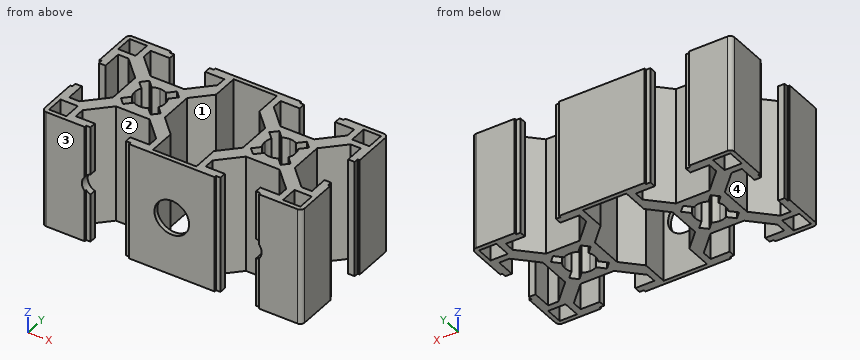
```python
from build123d import *

# Parameters (mm, degrees)
ESBO_O1_W                      = 4
ESBO_O1_H                      = 4
RESSALTO_EXTRUS_O1_DEPTH       = 27
PADR_OCIRCULAR1_COUNT          = 4
PADR_O_LINEAR1_COUNT           = 2
PADR_O_LINEAR1_PITCH           = 30
PADR_O_LINEAR1_COPY_1_SKETCH_W = 4
PADR_O_LINEAR1_COPY_1_SKETCH_H = 4
PADR_O_LINEAR1_COPY_1_DEPTH    = 27
PADR_O_LINEAR1_COPY_2_SKETCH_W = 4
PADR_O_LINEAR1_COPY_2_SKETCH_H = 4
PADR_O_LINEAR1_COPY_2_DEPTH    = 27
PADR_O_LINEAR1_COPY_3_SKETCH_W = 4
PADR_O_LINEAR1_COPY_3_SKETCH_H = 4
PADR_O_LINEAR1_COPY_3_DEPTH    = 27
ESBO_O4_W                      = 10
ESBO_O4_H                      = 28
CORTE_EXTRUS_O1_DEPTH          = 55.580216196
FILETE1_R                      = 1
SKETCH1_R                      = 2.5
SKETCH1_R_2                    = 4
CUT_EXTRUDE1_DEPTH             = 6


with BuildPart() as part:
    # Esboço1 → Ressalto-extrusão1 (new body)
    with BuildSketch(Plane.XY):
        with BuildLine():
            ThreePointArc((-1.664601464, 3.078815026), (-0.858529967, 3.393070335), (0, 3.5))
            Line((0, 3.5), (0, 6))
            Line((0, 6), (-3.878679656, 6))
            Line((-3.878679656, 6), (-8.5, 10.621320344))
            Line((-8.5, 10.621320344), (-8.5, 13))
            Line((-8.5, 13), (-4.1, 13))
            Line((-4.1, 13), (-4.1, 14.5))
            Line((-4.1, 14.5), (-5.1, 14.5))
            Line((-5.1, 14.5), (-5.1, 15))
            Line((-5.1, 15), (-15, 15))
            Line((-15, 15), (-15, 5.1))
            Line((-15, 5.1), (-14.5, 5.1))
            Line((-14.5, 5.1), (-14.5, 4.1))
            Line((-14.5, 4.1), (-13, 4.1))
            Line((-13, 4.1), (-13, 8.5))
            Line((-13, 8.5), (-10.621320344, 8.5))
            Line((-10.621320344, 8.5), (-6, 3.878679656))
            Line((-6, 3.878679656), (-6, 0))
            Line((-6, 0), (-3.5, 0))
            ThreePointArc((-3.5, 0), (-3.393070335, 0.858529967), (-3.078815026, 1.664601464))
            Line((-3.078815026, 1.664601464), (-4.596194078, 3.181980515))
            Line((-4.596194078, 3.181980515), (-3.181980515, 4.596194078))
            Line((-3.181980515, 4.596194078), (-1.664601464, 3.078815026))
        make_face()
        with Locations((-12, 12)):
            Rectangle(ESBO_O1_W, ESBO_O1_H, mode=Mode.SUBTRACT)
    ressalto_extrus_o1 = extrude(amount=RESSALTO_EXTRUS_O1_DEPTH)

    # PadrãoCircular1: Ressalto-extrusão1 ×4 about axis
    padr_ocircular1_axis = Axis((0, 0, 0), (0, 0, 1))
    for i in range(1, PADR_OCIRCULAR1_COUNT):
        add(ressalto_extrus_o1.rotate(padr_ocircular1_axis, i * 360 / PADR_OCIRCULAR1_COUNT))

    # Padrão linear1: Ressalto-extrusão1 ×2
    with Locations(*[(i * PADR_O_LINEAR1_PITCH, 0, 0) for i in range(1, PADR_O_LINEAR1_COUNT)]):
        add(ressalto_extrus_o1)

    # Padrão linear1 copy 1 sketch → Padrão linear1 copy 1 (add)
    with BuildSketch(Plane(origin=(30, 0, 0), x_dir=(0, 1, 0), z_dir=(0, 0, 1))):
        with BuildLine():
            ThreePointArc((-1.664601464, 3.078815026), (-0.858529967, 3.393070335), (0, 3.5))
            Line((0, 3.5), (0, 6))
            Line((0, 6), (-3.878679656, 6))
            Line((-3.878679656, 6), (-8.5, 10.621320344))
            Line((-8.5, 10.621320344), (-8.5, 13))
            Line((-8.5, 13), (-4.1, 13))
            Line((-4.1, 13), (-4.1, 14.5))
            Line((-4.1, 14.5), (-5.1, 14.5))
            Line((-5.1, 14.5), (-5.1, 15))
            Line((-5.1, 15), (-15, 15))
            Line((-15, 15), (-15, 5.1))
            Line((-15, 5.1), (-14.5, 5.1))
            Line((-14.5, 5.1), (-14.5, 4.1))
            Line((-14.5, 4.1), (-13, 4.1))
            Line((-13, 4.1), (-13, 8.5))
            Line((-13, 8.5), (-10.621320344, 8.5))
            Line((-10.621320344, 8.5), (-6, 3.878679656))
            Line((-6, 3.878679656), (-6, 0))
            Line((-6, 0), (-3.5, 0))
            ThreePointArc((-3.5, 0), (-3.393070335, 0.858529967), (-3.078815026, 1.664601464))
            Line((-3.078815026, 1.664601464), (-4.596194078, 3.181980515))
            Line((-4.596194078, 3.181980515), (-3.181980515, 4.596194078))
            Line((-3.181980515, 4.596194078), (-1.664601464, 3.078815026))
        make_face()
        with Locations((-12, 12)):
            Rectangle(PADR_O_LINEAR1_COPY_1_SKETCH_W, PADR_O_LINEAR1_COPY_1_SKETCH_H, mode=Mode.SUBTRACT)
    extrude(amount=PADR_O_LINEAR1_COPY_1_DEPTH)

    # Padrão linear1 copy 2 sketch → Padrão linear1 copy 2 (add)
    with BuildSketch(Plane(origin=(30, 0, 0), x_dir=(-1, 0, 0), z_dir=(0, 0, 1))):
        with BuildLine():
            ThreePointArc((-1.664601464, 3.078815026), (-0.858529967, 3.393070335), (0, 3.5))
            Line((0, 3.5), (0, 6))
            Line((0, 6), (-3.878679656, 6))
            Line((-3.878679656, 6), (-8.5, 10.621320344))
            Line((-8.5, 10.621320344), (-8.5, 13))
            Line((-8.5, 13), (-4.1, 13))
            Line((-4.1, 13), (-4.1, 14.5))
            Line((-4.1, 14.5), (-5.1, 14.5))
            Line((-5.1, 14.5), (-5.1, 15))
            Line((-5.1, 15), (-15, 15))
            Line((-15, 15), (-15, 5.1))
            Line((-15, 5.1), (-14.5, 5.1))
            Line((-14.5, 5.1), (-14.5, 4.1))
            Line((-14.5, 4.1), (-13, 4.1))
            Line((-13, 4.1), (-13, 8.5))
            Line((-13, 8.5), (-10.621320344, 8.5))
            Line((-10.621320344, 8.5), (-6, 3.878679656))
            Line((-6, 3.878679656), (-6, 0))
            Line((-6, 0), (-3.5, 0))
            ThreePointArc((-3.5, 0), (-3.393070335, 0.858529967), (-3.078815026, 1.664601464))
            Line((-3.078815026, 1.664601464), (-4.596194078, 3.181980515))
            Line((-4.596194078, 3.181980515), (-3.181980515, 4.596194078))
            Line((-3.181980515, 4.596194078), (-1.664601464, 3.078815026))
        make_face()
        with Locations((-12, 12)):
            Rectangle(PADR_O_LINEAR1_COPY_2_SKETCH_W, PADR_O_LINEAR1_COPY_2_SKETCH_H, mode=Mode.SUBTRACT)
    extrude(amount=PADR_O_LINEAR1_COPY_2_DEPTH)

    # Padrão linear1 copy 3 sketch → Padrão linear1 copy 3 (add)
    with BuildSketch(Plane(origin=(30, 0, 0), x_dir=(0, -1, 0), z_dir=(0, 0, 1))):
        with BuildLine():
            ThreePointArc((-1.664601464, 3.078815026), (-0.858529967, 3.393070335), (0, 3.5))
            Line((0, 3.5), (0, 6))
            Line((0, 6), (-3.878679656, 6))
            Line((-3.878679656, 6), (-8.5, 10.621320344))
            Line((-8.5, 10.621320344), (-8.5, 13))
            Line((-8.5, 13), (-4.1, 13))
            Line((-4.1, 13), (-4.1, 14.5))
            Line((-4.1, 14.5), (-5.1, 14.5))
            Line((-5.1, 14.5), (-5.1, 15))
            Line((-5.1, 15), (-15, 15))
            Line((-15, 15), (-15, 5.1))
            Line((-15, 5.1), (-14.5, 5.1))
            Line((-14.5, 5.1), (-14.5, 4.1))
            Line((-14.5, 4.1), (-13, 4.1))
            Line((-13, 4.1), (-13, 8.5))
            Line((-13, 8.5), (-10.621320344, 8.5))
            Line((-10.621320344, 8.5), (-6, 3.878679656))
            Line((-6, 3.878679656), (-6, 0))
            Line((-6, 0), (-3.5, 0))
            ThreePointArc((-3.5, 0), (-3.393070335, 0.858529967), (-3.078815026, 1.664601464))
            Line((-3.078815026, 1.664601464), (-4.596194078, 3.181980515))
            Line((-4.596194078, 3.181980515), (-3.181980515, 4.596194078))
            Line((-3.181980515, 4.596194078), (-1.664601464, 3.078815026))
        make_face()
        with Locations((-12, 12)):
            Rectangle(PADR_O_LINEAR1_COPY_3_SKETCH_W, PADR_O_LINEAR1_COPY_3_SKETCH_H, mode=Mode.SUBTRACT)
    extrude(amount=PADR_O_LINEAR1_COPY_3_DEPTH)

    # Esboço4 → Corte-extrusão1 (cut, through all)
    with BuildSketch(Plane(origin=(0, 0, 0), x_dir=(-1, 0, 0), z_dir=(0, 0, -1))):
        with Locations((-15, 0)):
            Rectangle(ESBO_O4_W, ESBO_O4_H)
    extrude(amount=-CORTE_EXTRUS_O1_DEPTH, mode=Mode.SUBTRACT)

    # Filete1
    filete1_edges = [part.edges().sort_by_distance(p)[0] for p in [
        (45, -15, 13.5),
        (45, 15, 13.5),
        (-15, 15, 13.5),
        (-15, -15, 13.5),
    ]]
    fillet(filete1_edges, radius=FILETE1_R)

    # Sketch1 → Cut-Extrude1 (cut)
    with BuildSketch(Plane.XZ.offset(15)):
        with Locations((33.25, 13.5)):
            Circle(SKETCH1_R)
        with Locations((-3.25, 13.5)):
            Circle(SKETCH1_R)
        with Locations(Location((15, 13.5, 0), (0, 0, 270))):
            Circle(SKETCH1_R_2)
    extrude(amount=-CUT_EXTRUDE1_DEPTH, mode=Mode.SUBTRACT)


solid = part.part
```
Work out the finished part from the listing and answer in its coordinate system (mm). Face numbers are marked on the shaded views. A direction names the side the tool comes from. Coordinates: 2 decimals unless noted, no trailing zeros. Write each loop counter-clockwise with the first axis right and the second up, starting at its lowest first coordinate (ties: lowest second). Pieces come first, ordered by that corner, then holes.
Q1. A cutting plane is placed at B-B, the plane y = -11.25. Give the vertices of the cut face in (x, z).
Q2. A cutting plane is placed at D-D, the plane y = -0.75. Give the vertices of the cut face in (x, z).
Q3. Which of the six approach directions +Z, -Z, +X, -X, +Y, -Y give full straight-line access (tool end or side, diameter ignored) to the marked faces 1, 2, 3 and 4?
Q4. A cutting plane is placed at C-C, the plane x = 7. Give the vertices of the cut face in (y, z).
Q5. A cutting plane is placed at A-A, the plane x = 15. Give the vertices of the cut face in (y, z), then the cut area to 3 significant figures.
Q6. Each of these flat-tipped pins is pushed along its axis until it touches: pin 1 Ø3 at (y, z) = (2.5, 6) entering from +X; pin 2 Ø2 at (y, z) = (4, 22.5) entering from -X; pin 3 Ø0.5 at (x, z) = (34.5, 6.5) entering from -Y. Where does it stop, or does it pass through?
Q7. Find the intervals of material crossed by line 1 (Y direction, x = -12, z = 25); line 2 (X direction, y = -13.25, z = 10.75); line 3 (X direction, y = -9.75, z = 6.25), in increasing order.
Findings below:
1. outline: (-15, 0) - (-14, 0) - (-14, 27) - (-15, 27) - close; (-10, 0) - (-8.5, 0) - (-8.5, 27) - (-10, 27) - close; (8.5, 0) - (10, 0) - (10, 27) - (8.5, 27) - close; (20, 0) - (21.5, 0) - (21.5, 27) - (20, 27) - close; (38.5, 0) - (40, 0) - (40, 27) - (38.5, 27) - close; (44, 0) - (45, 0) - (45, 27) - (44, 27) - close
2. outline: (-6, 0) - (-3.42, 0) - (-3.42, 27) - (-6, 27) - close; (3.42, 0) - (6, 0) - (6, 27) - (3.42, 27) - close; (24, 0) - (26.58, 0) - (26.58, 27) - (24, 27) - close; (33.42, 0) - (36, 0) - (36, 27) - (33.42, 27) - close
3. face 1: +Z, -Z
3. face 2: +Z, -Z, -Y
3. face 3: +Z, -Z, +X, -X, -Y
3. face 4: +Z, -Z, -X
4. outline: (-15, 0) - (-13, 0) - (-13, 27) - (-15, 27) - close; (-9.12, 0) - (-4.88, 0) - (-4.88, 27) - (-9.12, 27) - close; (4.88, 0) - (9.12, 0) - (9.12, 27) - (4.88, 27) - close; (13, 0) - (15, 0) - (15, 27) - (13, 27) - close
5. outline: (-15, 0) - (-14, 0) - (-14, 9.5) - (-15, 9.5) - close; (-15, 17.5) - (-14, 17.5) - (-14, 27) - (-15, 27) - close; (14, 0) - (15, 0) - (15, 27) - (14, 27) - close
5. area: 46.0 mm2
6. pin 1: stops at x = 36.12
6. pin 2: stops at x = -14.5
6. pin 3: stops at y = -14.5
7. line 1: y = -15 to -14, -10 to -8.5, 8.5 to 10, 14 to 15
7. line 2: x = -15 to -14, -10 to -4.1, 4.1 to 10, 20 to 25.9, 34.1 to 40, 44 to 45
7. line 3: x = -15 to -7.63, 7.63 to 10, 20 to 22.37, 37.63 to 45
